The model under review builds one solid part; all positions refer to its coordinate system, in mm. A direction names the side the tool comes from. Coordinates: 2 decimals unless noted, no trailing zeros. Loops run counter-clockwise (first coordinate to the right, second up) from the corner with the lowest first, then second, coordinate; pieces in that order, holes last. Notation, with made-up numbers: (-23, -23.75) - (15, -23.75) arc R27 ccw to (15, 4.25) - close; hole circle Ø8 at (0, 71). An arc over 180 degrees is marked (long way). Use a Markdown table: item, result. Add a question column.
1) To check wall thickness, follow L1, parallel to Z at x = 23, y = 4.25; L2, parallel to Y at x = -48, z = -11 (3 decimals); L3, parallel to Z at x = 0, y = 1. State the ranges of each line that lie inside material, in increasing order. Write a range as [from, to].
2) Add section A-A, the plane y = 6. Give the boundary of the cut face in (x, z).
3) Clearance check with flat-ended pins moving along their axes: pin 1 (12 mm diameter, centred on x = 35.5, z = -49.5, fed in from +Y) (3 decimals); pin 2 (1.5 mm diameter, centred on y = -1.5, z = -18, fed in from +X); pin 3 (4 mm diameter, centred on x = 13, y = 1.5, fed in from +Z). State where each tip first meets the part, or that it passes through.
4) The part is to be moulded in two halves that separate along Z. For faces 5 (the cylindrical face through (-71.987, 11.301, -40.707)), 6 (the flat face through (55.291, -0.044, -31.306)), 7 (the cylindrical face through (-43.22, 11.34, 4.47)), say which applies: pulls with the +Z half, pulls with the -Z half, needs draft (parallel to the pull), parting line crosses it, or undercut.
5) Add section C-C, the plane z = -16. Give the boundary of the cut face in (x, y) (3 decimals).
6) For faces 1 (the flat face through (11, 6, -6.35)), 2 (the flat face through (-45.28, 6.31, 5.45)), 3 (the flat face through (1, 6, -57.15)), 4 (the cylindrical face through (-75.41, 11.3, -44.22)), list the 3-axis set-ups (+Z, -Z, +X, -X, +Y, -Y) from which the entire face can be reached by the end or side of a thin tool; tool diameter is ignored.
7) Add section B-B, the plane x = 25. Give the boundary of the cut face in (y, z) (3 decimals), and give its area (3 significant figures).
```python
from build123d import *

# Parameters (mm, degrees)
SKETCH1_W               = 114.3
SKETCH1_H               = 6.35
BOSS_EXTRUDE1_DEPTH     = 63.5
SKETCH2_W               = 114.3
SKETCH2_H               = 6.35
BOSS_EXTRUDE2_DEPTH     = 8.89
CUT_EXTRUDE1_DEPTH      = 64.5
CUT_EXTRUDE2_DEPTH      = 13.065
CUT_EXTRUDE2_DEPTH_BACK = 4.175
BOSS_EXTRUDE4_DEPTH     = 3.175
BOSS_EXTRUDE5_DEPTH     = 8.89
FILLET1_R               = 2.54
CUT_EXTRUDE3_DEPTH      = 93.267614143


with BuildPart() as part:
    # Sketch1 → Boss-Extrude1 (new body)
    with BuildSketch(Plane.XY):
        Rectangle(SKETCH1_W, SKETCH1_H)
    extrude(amount=-BOSS_EXTRUDE1_DEPTH)

    # Sketch2 → Boss-Extrude2 (add)
    with BuildSketch(Plane(origin=(0, 3.175, 0), x_dir=(1, 0, 0), z_dir=(0, 1, 0))):
        with Locations((0, 60.325)):
            Rectangle(SKETCH2_W, SKETCH2_H)
        with Locations((0, 3.175)):
            Rectangle(SKETCH2_W, SKETCH2_H)
    extrude(amount=BOSS_EXTRUDE2_DEPTH)

    # Sketch3 → Cut-Extrude1 (cut, through all)
    with BuildSketch(Plane.XY):
        Polygon((57.15, 3.175), (41.752068321, 12.065), (48.527437664, 23.800283942), (66.675, 13.322783942), (57.15, -3.175), (56.233456448, -4.7625), (53.483825791, -3.175), align=None)
    extrude(amount=-CUT_EXTRUDE1_DEPTH, mode=Mode.SUBTRACT)

    # Sketch5 → Cut-Extrude2 (cut, two sides)
    with BuildSketch(Plane(origin=(0, 0, 0), x_dir=(1, 0, 0), z_dir=(0, 1, 0))) as cut_extrude2_sk:
        Polygon((-57.15, 63.5), (-30.847438789, 0), (-57.15, 0), align=None)
    extrude(amount=CUT_EXTRUDE2_DEPTH, mode=Mode.SUBTRACT)
    extrude(cut_extrude2_sk.sketch, amount=-CUT_EXTRUDE2_DEPTH_BACK, mode=Mode.SUBTRACT)

    # Sketch9 → Boss-Extrude4 (add, symmetric)
    with BuildSketch(Plane(origin=(0, 0, 0), x_dir=(1, 0, 0), z_dir=(0, 1, 0))):
        Polygon((-30.847438789, 0), (-57.15, 63.5), (-97.833550078, 22.816449922), (-52.932269473, -22.084830683), align=None)
    extrude(amount=BOSS_EXTRUDE4_DEPTH, both=True)

    # Sketch11 → Boss-Extrude5 (add)
    with BuildSketch(Plane(origin=(0, 3.175, 0), x_dir=(1, 0, 0), z_dir=(0, 1, 0))):
        Polygon((-57.15, 63.5), (-97.833550078, 22.816449922), (-93.343422018, 18.326321861), (-54.519743879, 57.15), align=None)
        Polygon((-33.47769491, 6.35), (-57.422397533, -17.594702623), (-52.932269473, -22.084830683), (-30.847438789, 0), align=None)
    extrude(amount=BOSS_EXTRUDE5_DEPTH)

    # Fillet1
    fillet1_edges = [part.edges().sort_by_distance(p)[0] for p in [
        (-41.889854131, 12.065, 11.042415342),
        (5.452314766, 12.065, 0),
        (4.137186705, 12.065, -6.35),
        (-45.450046222, 12.065, 5.622351311),
        (-73.931582948, 12.065, -37.738160931),
        (-6.383837779, 12.065, -57.15),
        (-7.69896584, 12.065, -63.5),
        (-77.491775039, 12.065, -43.158224961),
    ]]
    fillet(fillet1_edges, radius=FILLET1_R)

    # Sketch12 → Cut-Extrude3 (cut, through all)
    with BuildSketch(Plane(origin=(-15.423719395, 0, -15.423719395), x_dir=(0.707106781, 0, -0.707106781), z_dir=(0.707106781, 0, 0.707106781))):
        Polygon((-53.045100225, 3.175), (-45.267970292, -3.175), (-53.300155549, -13.012377699), (-72.974910948, 3.051992814), (-56.910540434, 22.726748213), (-45.012914969, 13.012377699), align=None)
    extrude(amount=-CUT_EXTRUDE3_DEPTH, mode=Mode.SUBTRACT)


solid = part.part
```
From the geometry:
| question | item | result |
|---|---|---|
| 1 | L1 | z = [-63.5, -57.15], [-6.35, 0] |
| 1 | L2 | y = [-3.175, 3.175] |
| 1 | L3 | z = [-63.5, 0] |
| 2 | outline | (-96.2, -24.45) - (-57.15, -63.5) - (52.26, -63.5) - (52.26, -57.15) - (-54.52, -57.15) - (-91.71, -19.96) - close; (-55.79, 15.96) - (-33.48, -6.35) - (52.26, -6.35) - (52.26, 0) - (-30.85, 0) - (-51.3, 20.45) - close |
| 3 | pin 1 | stops at y = 3.175 |
| 3 | pin 2 | stops at x = 54.88 |
| 3 | pin 3 | stops at z = 0 |
| 4 | face 5 | pulls with the +Z half |
| 4 | face 6 | needs draft |
| 4 | face 7 | undercut |
| 5 | outline | (-91.017, 3.175) - (-80.019, -3.175) - (53.484, -3.175) - (57.15, 3.175) - close |
| 6 | face 1 | +X, -X, +Y |
| 6 | face 2 | -X, +Y |
| 6 | face 3 | +X, +Y |
| 6 | face 4 | -Z, -X, +Y |
| 7 | outline | (-3.175, -63.5) - (9.525, -63.5) arc R2.54 ccw to (12.065, -60.96) - (12.065, -59.69) arc R2.54 ccw to (9.525, -57.15) - (3.175, -57.15) - (3.175, -6.35) - (9.525, -6.35) arc R2.54 ccw to (12.065, -3.81) - (12.065, -2.54) arc R2.54 ccw to (9.525, 0) - (-3.175, 0) - close |
| 7 | area | 511 mm^2 |
